Input: part model. Units: mm. Frame: model coordinates. A direction names the side the tool comes from. Coordinates: 2 decimals unless noted, no trailing zeros. Loops run counter-clockwise (first coordinate to the right, second up) from the corner with the lowest first, then second, coordinate; pieces in that order, holes last.
Autodesk Inventor part; units mm, degrees
ref_plane "YZ Plane" through (0, 0, 0) normal (1, 0, 0) x (0, 1, 0)
ref_plane "XZ Plane" through (0, 0, 0) normal (0, 1, 0) x (-1, 0, 0)
ref_plane "XY Plane" through (0, 0, 0) normal (0, 0, 1) x (1, 0, 0)
sketch "Sketch1" plane through (0, 0, 0) normal (0, 1, 0) x (-1, 0, 0)
  line L0 (0, 0) -> (40, 0)
  line L1 (40, 0) -> (40, -40)
  line L2 (40, -40) -> (0, -40)
  line L3 (0, -40) -> (0, 0)
  dimension "d0" = 40
  dimension "d1" = 40
extrude "Extrusion1" add sketch "Sketch1" along normal blind 10
sketch "Sketch2" plane through (0, 10, 0) normal (0, 1, 0) x (1, 0, 0)
  circle A0 centre (-20, 20) radius 4
  point P0 (0, 0)
  dimension "d4" = 8
extrude "Extrusion2" add sketch "Sketch2" along normal blind 20
sketch "Sketch3" plane through (-20, 30, -20) normal (0, 1, 0) x (1, 0, 0)
  line L0 (2.6327, 1.6155) -> (2.7154, -1.4722)
  line L1 (2.7154, -1.4722) -> (0.0827, -3.0877)
  line L2 (0.0827, -3.0877) -> (-2.6327, -1.6155)
  line L3 (-2.6327, -1.6155) -> (-2.7154, 1.4722)
  line L4 (-2.7154, 1.4722) -> (-0.0827, 3.0877)
  line L5 (-0.0827, 3.0877) -> (2.6327, 1.6155)
  point P0 (20, -20)
  point P1 (0, 0)
  dimension "d7" = 5.35
extrude "Extrusion3" cut sketch "Sketch3" against normal blind 2.5
sketch "Sketch4" plane through (-20, 27.5, -20) normal (0, 1, 0) x (1, 0, 0)
  circle A0 centre (0, 0) radius 1.375
  point P0 (20, -20)
  dimension "d10" = 2.75
extrude "Extrusion4" cut sketch "Sketch4" against normal blind 2.5
properties part number "YMount_Belt"
Item 1: Section query A-A (z = -20). Output: boundary loops of the cut face in (x, y) (3 decimals).
Result:
outline: (-40, 0) - (0, 0) - (0, 10) - (-16, 10) - (-16, 30) - (-17.324, 30) - (-17.324, 27.5) - (-18.625, 27.5) - (-18.625, 25) - (-21.375, 25) - (-21.375, 27.5) - (-22.676, 27.5) - (-22.676, 30) - (-24, 30) - (-24, 10) - (-40, 10) - close
Item 2: Section query D-D (x = -22). Output: boundary loops of the cut face in (y, z), then the cut area to 3 significant figures.
Result:
outline: (0, -40) - (10, -40) - (10, -23.46) - (30, -23.46) - (30, -21.91) - (27.5, -21.91) - (27.5, -18.04) - (30, -18.04) - (30, -16.54) - (10, -16.54) - (10, 0) - (0, 0) - close
area: 529 mm2
Item 3: Mould query, pull axis Z, two halves, no side actions, for faces 1 (the face through (-20, 5, 0)), 2 (the face through (-21.417, 28.768, -22.269)), 3 (the face through (-24.2, 10, -19.7)). Classes: +Z half, -Z half, draft (parallel to the pull), parting line (faces both ways), or undercut.
Result:
face 1: +Z half
face 2: undercut
face 3: draft
Item 4: Line query: L1, parallel to Z at x = -20, y = 26.55 (3 decimals); L2, parallel to Y at x = -29.5, z = -11.5. Output: solid intervals per line, ascending.
Result:
L1: z = -24 to -21.375, -18.625 to -16
L2: y = 0 to 10
Item 5: Section query B-B (y = 23). Output: boundary loops of the cut face in (x, z), then the cut area to 3 significant figures.
Result:
outline: circle Ø8 at (-20, -20)
area: 50.3 mm2
Item 6: Contact query for flat-ended pins moving along their axis: P1, Ø10, axis at x = -31, y = 17, coming from the -Z side; P2, Ø2, axis at x = -20.5, z = -20, coming from the +Y side; P3, Ø12, axis at x = -10, z = -17.5, coming from the +Y side; P4, Ø10, axis at y = 17, z = -20, coming from the +X side. Output: stop coordinate, or through.
Result:
P1: passes through
P2: stops at y = 27.5
P3: stops at y = 10
P4: stops at x = -16
Item 7: Section query C-C (x = -26). Output: boundary loops of the cut face in (y, z), then the cut area to 3 significant figures.
Result:
outline: (0, -40) - (10, -40) - (10, 0) - (0, 0) - close
area: 400 mm2
Item 8: Reachability of faces 4 (the face through (-40, 5, -20)), 5 (the face through (-21.26, 28.77, -17.64)) from +Z, -Z, +X, -X, +Y, -Y: full face, straight path, thin tool, end or side. Return the list, or none.
Result:
face 4: +Z, -Z, -X, +Y, -Y
face 5: +Y
